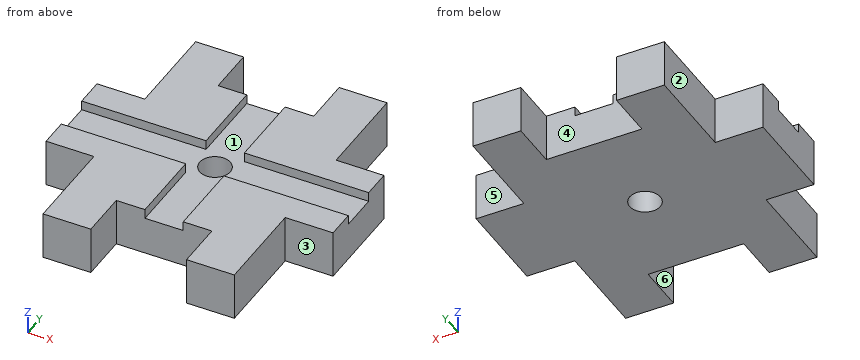
Autodesk Inventor part; units mm, degrees
ref_plane "YZ Plane" through (0, 0, 0) normal (1, 0, 0) x (0, 1, 0)
ref_plane "XZ Plane" through (0, 0, 0) normal (0, 1, 0) x (-1, 0, 0)
ref_plane "XY Plane" through (0, 0, 0) normal (0, 0, 1) x (1, 0, 0)
sketch "スケッチ1" plane through (0, 0, 0) normal (0, 0, 1) x (1, 0, 0)
  line L0 (-15, -15) -> (15, -15)
  line L1 (15, -15) -> (15, 15)
  line L2 (15, 15) -> (-15, 15)
  line L3 (-15, 15) -> (-15, -15)
  line L4 (-15, -15) -> (15, 15) construction
  line L5 (15, -15) -> (-15, 15) construction
  point P0 (0, 0)
  dimension "d2" = 30
  dimension "d3" = 30
extrude "押し出し1" add sketch "スケッチ1" along normal blind 5
sketch "スケッチ2" plane through (0, 0, 5) normal (0, 0, 1) x (1, 0, 0)
  line L0 (-15, 15) -> (-10, 15)
  line L1 (-10, 15) -> (-10, 5)
  line L2 (-10, 5) -> (-15, 5)
  line L3 (-15, 5) -> (-15, 15)
  line L4 (-15, -15) -> (-10, -15)
  line L5 (-10, -15) -> (-10, -5)
  line L6 (-10, -5) -> (-15, -5)
  line L7 (-15, -5) -> (-15, -15)
  line L8 (15, 15) -> (-15, 15)
  line L9 (10, 15) -> (15, 15)
  line L10 (15, 15) -> (15, 5)
  line L11 (15, 5) -> (10, 5)
  line L12 (10, 5) -> (10, 15)
  line L13 (15, -15) -> (10, -15)
  line L14 (10, -15) -> (10, -5)
  line L15 (10, -5) -> (15, -5)
  line L16 (15, -5) -> (15, -15)
  line L17 (-5, 15) -> (5, 15)
  line L18 (5, 15) -> (5, 10)
  line L19 (5, 10) -> (-5, 10)
  line L20 (-5, 10) -> (-5, 15)
  line L21 (-15, -15) -> (15, -15)
  line L22 (-5, -15) -> (5, -15)
  line L23 (5, -15) -> (5, -10)
  line L24 (5, -10) -> (-5, -10)
  line L25 (-5, -10) -> (-5, -15)
  point P0 (0, 0)
  dimension "d6" = 10
  dimension "d7" = 10
  dimension "d8" = 5
  dimension "d9" = 10
  dimension "d10" = 5
  dimension "d11" = 5
  dimension "d12" = 10
  dimension "d13" = 10
  dimension "d14" = 5
  dimension "d15" = 5
  dimension "d16" = 5
extrude "押し出し2" cut sketch "スケッチ2" against normal blind 5
sketch "スケッチ4" plane through (0, 0, 5) normal (0, 0, 1) x (1, 0, 0)
  line L0 (-20.2222, 2) -> (20.2222, 2)
  line L1 (20.2222, 2) -> (20.2222, -2)
  line L2 (20.2222, -2) -> (-20.2222, -2)
  line L3 (-20.2222, -2) -> (-20.2222, 2)
  line L4 (-20.2222, 2) -> (20.2222, -2) construction
  line L5 (20.2222, 2) -> (-20.2222, -2) construction
  line L6 (-2, 16.5333) -> (2, 16.5333)
  line L7 (2, 16.5333) -> (2, -16.5333)
  line L8 (2, -16.5333) -> (-2, -16.5333)
  line L9 (-2, -16.5333) -> (-2, 16.5333)
  line L10 (-2, 16.5333) -> (2, -16.5333) construction
  line L11 (2, 16.5333) -> (-2, -16.5333) construction
  point P0 (0, 0)
  dimension "d19" = 4
  dimension "d20" = 4
extrude "押し出し3" cut sketch "スケッチ4" against normal blind 1
sketch "スケッチ5" plane through (0, 0, 5) normal (0, 0, 1) x (1, 0, 0)
  circle A0 centre (0, 0) radius 1.6
  dimension "d23" = 3.2
extrude "押し出し4" cut sketch "スケッチ5" against normal up to next
sketch "スケッチ7" plane through (0, 0, 5) normal (0, 0, 1) x (1, 0, 0)
  line L0 (-10, 5) -> (-11.0607, 6.0607) construction
  circle A0 centre (-11.0607, 6.0607) radius 1.5
  line L1 (-10, 5) -> (-15, 5) construction
  line L2 (-5, 10) -> (-3.8771, 10) construction
  line L3 (-2, 10) -> (-5, 10)
  line L4 (-5, 10) -> (-3.9393, 11.0607) construction
  circle A1 centre (-3.9393, 11.0607) radius 1.5
  line L5 (0, 0) -> (-3.2296, 0)
  line L6 (0, 0) -> (0, 2.4653)
  line L7 (10, 5) -> (11.0607, 6.0607) construction
  circle A2 centre (11.0607, 6.0607) radius 1.5
  line L8 (10, 5) -> (15, 5) construction
  line L9 (5, 10) -> (3.8771, 10) construction
  line L10 (2, 10) -> (5, 10)
  line L11 (5, 10) -> (3.9393, 11.0607) construction
  circle A3 centre (3.9393, 11.0607) radius 1.5
  line L12 (-10, -5) -> (-11.0607, -6.0607) construction
  circle A4 centre (-11.0607, -6.0607) radius 1.5
  line L13 (-10, -5) -> (-15, -5) construction
  line L14 (-5, -10) -> (-3.8771, -10) construction
  line L15 (-2, -10) -> (-5, -10)
  line L16 (-5, -10) -> (-3.9393, -11.0607) construction
  circle A5 centre (-3.9393, -11.0607) radius 1.5
  line L17 (10, -5) -> (11.0607, -6.0607) construction
  circle A6 centre (11.0607, -6.0607) radius 1.5
  line L18 (10, -5) -> (15, -5) construction
  line L19 (5, -10) -> (3.8771, -10) construction
  line L20 (2, -10) -> (5, -10)
  line L21 (5, -10) -> (3.9393, -11.0607) construction
  circle A7 centre (3.9393, -11.0607) radius 1.5
  dimension "d27" = 3
  dimension "d29" = 3
  dimension "d26" = 45
  dimension "d28" = 45
extrude "押し出し5" [suppressed]
properties part number "piece_1"
Check sheet for the modelled part. Datum: model origin and axes. Units: mm. Face numbers are marked on the shaded views. A direction names the side the tool comes from. Round coordinates to 2 decimals unless told otherwise and drop trailing zeros. Write each loop counter-clockwise with the first axis right and the second up, starting at its lowest first coordinate (ties: lowest second). Pieces come first, ordered by that corner, then holes. Notation, with made-up numbers: (-34.75, 19.5) - (8.25, 19.5) arc R20 ccw to (8.25, 23.5) - close; hole circle Ø10 at (87.5, 28). An arc over 180 degrees is marked (long way). Return JSON: item names as keys, results as strings.
Q1. Depth check by flat-ended pin: P1, Ø1.5, axis at y = 12.5, z = 1.5, coming from the -X side; P2, Ø2.5, axis at y = 13.5, z = 2, coming from the +X side; P3, Ø3, axis at x = 0, y = 3, coming from the +Z side. Enter the tip coordinate at first touch or a pass-through.
Returned:
{"P1": "stops at x = -10", "P2": "stops at x = 10", "P3": "stops at z = 4"}
Q2. Scan lines: L1, parallel to X at y = -8.75, z = 4.15; L2, parallel to X at y = 12, z = 3.95; L3, parallel to X at y = 7, z = 3.8. Record each from-to range of solid material in increasing order. Write a range as from..to.
Returned:
{"L1": "x = -10..-2, 2..10", "L2": "x = -10..-5, 5..10", "L3": "x = -10..10"}
Q3. Cross-section at C-C (x = 6.25). Record the boundary of the cut face in (y, z), then the cut area to 3 significant figures.
Returned:
{"outline": "(-15, 0) - (15, 0) - (15, 5) - (2, 5) - (2, 4) - (-2, 4) - (-2, 5) - (-15, 5) - close", "area": "146 mm²"}
Q4. Cross-section at B-B (z = 1.8). Record the boundary of the cut face in (x, y).
Returned:
{"outline": "(-15, -5) - (-10, -5) - (-10, -15) - (-5, -15) - (-5, -10) - (5, -10) - (5, -15) - (10, -15) - (10, -5) - (15, -5) - (15, 5) - (10, 5) - (10, 15) - (5, 15) - (5, 10) - (-5, 10) - (-5, 15) - (-10, 15) - (-10, 5) - (-15, 5) - close; hole circle Ø3.2 at (0, 0)"}
Q5. Access from +Z, -Z, +X, -X, +Y, -Y to the whole of each face (thin tool, end or side, straight path). Record for the marked faces 4, 5 and 6.
Returned:
{"face 4": "+Z, -Z, +Y", "face 5": "+Z, -Z, +X, +Y", "face 6": "+Z, -Z, -Y"}
Q6. Cross-section at A-A (y = 0). Record the boundary of the cut face in (x, z), then the cut area to 3 significant figures.
Returned:
{"outline": "(-15, 0) - (-1.6, 0) - (-1.6, 4) - (-15, 4) - close; (1.6, 0) - (15, 0) - (15, 4) - (1.6, 4) - close", "area": "107 mm²"}
Q7. Draft check along X on the marked faces 1, 2 and 3. Enter one of: released by +X, released by -X, zero draft, split by the parting line, or undercut.
Returned:
{"face 1": "undercut", "face 2": "released by -X", "face 3": "zero draft"}
Q8. Cross-section at D-D (x = 0). Record the boundary of the cut face in (y, z).
Returned:
{"outline": "(-10, 0) - (-1.6, 0) - (-1.6, 4) - (-10, 4) - close; (1.6, 0) - (10, 0) - (10, 4) - (1.6, 4) - close"}
